from build123d import *

# Parameters (mm, degrees)
BOX003_W                  = 2.2
BOX003_H                  = 1.5
BOX003_DEPTH              = 1.5
BOX001_W                  = 5
BOX001_H                  = 7.8
BOX001_DEPTH              = 2.5
SKETCH006_R               = 0.5
SKETCH006_W               = 1.5
SKETCH006_H               = 1.5
PAD006_DEPTH              = 1.5
FUSION002_PITCH_ANGLE     = 90
FUSION002_PLACEMENT_ANGLE = -180
BOX002_W                  = 2.2
BOX002_H                  = 1.5
BOX002_DEPTH              = 1.5


with BuildPart() as cube002:
    # Box003 → Box003 (new body)
    with BuildSketch(Plane(origin=(-16.2, -8.005, 13.3), x_dir=(1, 0, 0), z_dir=(0, 0, 1))):
        with Locations((1.1, 0.75)):
            Rectangle(BOX003_W, BOX003_H)
    extrude(amount=BOX003_DEPTH)


with BuildPart() as cube:
    # Box001 → Box001 (new body)
    with BuildSketch(Plane(origin=(-14.25, -3.9, 1), x_dir=(1, 0, 0), z_dir=(0, 0, 1))):
        with Locations((2.5, 3.9)):
            Rectangle(BOX001_W, BOX001_H)
    extrude(amount=BOX001_DEPTH)


with BuildPart() as re:
    # Sketch006 → Pad006 (new body)
    with BuildSketch(Plane.XY):
        Polygon((-13, 8.504137), (14.28215, 8.504137), (14.28215, 6.5), (13, 6.5), (13, -6.5), (14.28215, -6.5), (14.28215, -8.504137), (-13, -8.504137), (-13, -3.9), (-14.250851, -3.9), (-14.250851, 3.9), (-13, 3.9), align=None)
        with Locations((-11.5, 7.004137)):
            Circle(SKETCH006_R, mode=Mode.SUBTRACT)
        with Locations((-11.5, -7.004137)):
            Circle(SKETCH006_R, mode=Mode.SUBTRACT)
        with Locations((11.5, 7.004137)):
            Circle(SKETCH006_R, mode=Mode.SUBTRACT)
        with Locations((11.5, 4.464137)):
            Circle(SKETCH006_R, mode=Mode.SUBTRACT)
        with Locations((11.5, -7.004137)):
            Circle(SKETCH006_R, mode=Mode.SUBTRACT)
        with Locations((11.5, -4.464137)):
            Circle(SKETCH006_R, mode=Mode.SUBTRACT)
        with Locations((-6.25, 7.254137)):
            Rectangle(SKETCH006_W, SKETCH006_H, mode=Mode.SUBTRACT)
        with Locations((-2.25, 7.25)):
            Rectangle(SKETCH006_W, SKETCH006_H, mode=Mode.SUBTRACT)
    extrude(amount=PAD006_DEPTH)

    # Fusion002: union Cube
    add(cube.part)


with BuildPart() as re_1:
    # Fusion002 pitch: moved
    add(re.part.rotate(Axis((0, 0, 0), (0, 1, 0)), FUSION002_PITCH_ANGLE))


with BuildPart() as re_2:
    # Fusion002 placement: moved
    add(re_1.part.moved(Location((-14, 0, 11.8))).rotate(Axis((-14, 0, 11.8), (0, 0, 1)), FUSION002_PLACEMENT_ANGLE))


with BuildPart() as obj1:
    # Box002 → Box002 (new body)
    with BuildSketch(Plane(origin=(-16.2, -8.005, 17.3), x_dir=(1, 0, 0), z_dir=(0, 0, 1))):
        with Locations((1.1, 0.75)):
            Rectangle(BOX002_W, BOX002_H)
    extrude(amount=BOX002_DEPTH)

    # Fusion003: union Cube002, Re
    add(cube002.part)
    add(re_2.part)


with BuildPart() as obj1_1:
    # Fusion003 placement: moved
    add(obj1.part.moved(Location((-4, 0, -1))))


solid = obj1_1.part
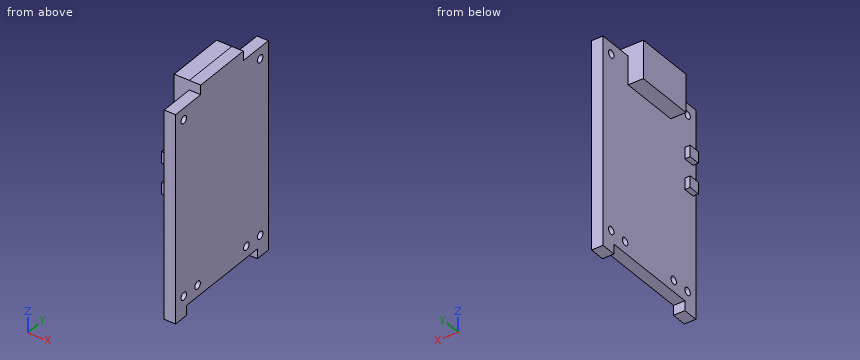
Could you check a few things on this model? Use its own coordinates, in mm. Give positions to 0.01 mm unless a question says otherwise; leave off trailing zeros. Loops run counter-clockwise (first coordinate to the right, second up) from the corner with the lowest first, then second, coordinate; pieces in that order, holes last. Notation, with made-up numbers: (-9, -37.75) -> (0, -37.75) arc R23 ccw to (0, -16.75) -> close; hole circle Ø2 at (30.25, 22). An arc over 180 degrees is marked (long way). Answer as CSV lines item,"result". Start each with the question number.
(1) If we section it at A-A on z = -0.7: Write out the boundary of the cut face in (x, y), then the cut area to 3 significant figures.
(2) I need wall thicknesses on probe 1 along Y at (x, z) = (-19.05, 22.3); probe 2 along Y at (x, z) = (-18.7, -0.7); probe 3 along Z at (x, y) = (-18.4, 7.25). Which ranges of each line are inside material? Lowest first, please.
(3) I'm going to push flat-ended pins straight in: pin 1 Ø0.8 at (x, y) = (-20, -7) entering from +Z; pin 2 Ø1 at (x, y) = (-20.5, 0.5) entering from -Z; pin 3 Ø0.8 at (x, y) = (-20, -7) entering from -Z; pin 4 Ø1 at (x, y) = (-20.5, 5) entering from +Z. Where does each tip first touch, or does it pass through?
(4) If we section it at D-D on x = -18.55: Count the separate pieces of the cut face and the enclosed holes in it, then the cut area to 3 significant figures.
(5) If we section it at B-B on z = 22.3: Write out the boundary of the cut face in (x, y).
Computed:
1,outline,"(-19.5, -8.5) -> (-18, -8.5) -> (-18, -7.5) -> (-19.5, -7.5) -> close; (-19.5, -6.5) -> (-18, -6.5) -> (-18, -4.96) -> (-19.5, -4.96) -> close; (-19.5, -3.96) -> (-18, -3.96) -> (-18, 3.96) -> (-19.5, 3.96) -> close; (-19.5, 4.96) -> (-18, 4.96) -> (-18, 6.5) -> (-19.5, 6.5) -> close; (-19.5, 7.5) -> (-18, 7.5) -> (-18, 8.5) -> (-19.5, 8.5) -> close"
1,area,"19.5 mm2"
2,probe 1,"y = -8.5 to -7.5, -6.5 to 6.5, 7.5 to 8.5"
2,probe 2,"y = -8.5 to -7.5, -6.5 to -4.96, -3.96 to 3.96, 4.96 to 6.5, 7.5 to 8.5"
2,probe 3,"z = -3.48 to -1.14, -0.26 to 21.86, 22.74 to 23.8"
3,pin 1,"stops at z = 17.8"
3,pin 2,"stops at z = 20.05"
3,pin 3,"stops at z = 12.3"
3,pin 4,"passes through"
4,separate pieces,"1"
4,enclosed holes,"8"
4,area,"452 mm2"
5,outline,"(-21.5, -3.9) -> (-19.5, -3.9) -> (-19.5, -6.5) -> (-18, -6.5) -> (-18, 6.5) -> (-19.5, 6.5) -> (-19.5, 3.9) -> (-21.5, 3.9) -> close; (-19.5, -8.5) -> (-18, -8.5) -> (-18, -7.5) -> (-19.5, -7.5) -> close; (-19.5, 7.5) -> (-18, 7.5) -> (-18, 8.5) -> (-19.5, 8.5) -> close"
